Input: part model. Units: mm. Frame: model coordinates. A direction names the side the tool comes from. Coordinates: 2 decimals unless noted, no trailing zeros. Loops run counter-clockwise (first coordinate to the right, second up) from the corner with the lowest first, then second, coordinate; pieces in that order, holes last. Notation, with made-up numbers: (35, -29.5) - (80, -29.5) arc R34 cw to (80, 2.5) - close; hole circle Ø4 at (-4, 82). An arc over 180 degrees is marked (long way). Answer as CSV lines item,"result". Start each with the question number.
```python
from build123d import *

# Parameters (mm, degrees)
SKETCH_2_W          = 380.47
SKETCH_2_H          = 189.04
EXTRUDE_1_DEPTH     = 3
SKETCH_3_W          = 368.48
SKETCH_3_H          = 177.01
EXTRUDE_2_DEPTH     = 11.5
SKETCH_4_W          = 352.48
SKETCH_4_H          = 161.01
CUT_EXTRUDE_1_DEPTH = 11.5


with BuildPart() as part:
    # 草图2 → 凸台-拉伸1 (new body)
    with BuildSketch(Plane.XY):
        with Locations((183.815306963, 88.27515573)):
            Rectangle(SKETCH_2_W, SKETCH_2_H)
    extrude(amount=EXTRUDE_1_DEPTH)

    # 草图3 → 凸台-拉伸2 (add)
    with BuildSketch(Plane.XY.offset(3)):
        with Locations((183.815306963, 88.27515573)):
            Rectangle(SKETCH_3_W, SKETCH_3_H)
    extrude(amount=EXTRUDE_2_DEPTH)

    # 草图4 → 切除-拉伸1 (cut)
    with BuildSketch(Plane.XY.offset(14.5)):
        with Locations((183.815306963, 88.27515573)):
            Rectangle(SKETCH_4_W, SKETCH_4_H)
    extrude(amount=-CUT_EXTRUDE_1_DEPTH, mode=Mode.SUBTRACT)


solid = part.part
```
Item 1: Set-up query: faces 1 (the flat face through (181, 176.78, 9)), 2 (the flat face through (181, 168.78, 9)), 3 (the flat face through (-0.425, 87, 9)). Return all of +Z, -Z, +X, -X, +Y, -Y with unobstructed straight access to the full face (end or side cutting, diameter ignored); none if empty.
Item 2: Section query C-C, the plane x = 66.5. Output: boundary loops of the cut face in (y, z).
Item 3: Draft query along X for faces 4 (the flat face through (368.055, 87, 9)), 5 (the flat face through (181, 7.77, 9)), 6 (the flat face through (183, 180, 3)). Return one class per face: pulls with the +X half, pulls with the -X half, needs draft (parallel to the pull), parting line crosses it, or undercut.
Item 4: Section query A-A, the plane z = 8.5. Output: boundary loops of the cut face in (x, y), and give its area (3 significant figures).
Item 5: Contact query for flat-ended pins moving along their axis: P1, Ø10, axis at x = 150.5, y = 66.5, coming from the +Z side; P2, Ø1.5, axis at y = 59.5, z = 6.5, coming from the +X side; P3, Ø6, axis at x = 233.5, z = 10.5, coming from the +Y side. Output: stop coordinate, or through.
Item 6: Material intervals for probe 1 along X at (y, z) = (19, 4.5); probe 2 along Y at (x, z) = (195.5, 3.25); probe 3 along Z at (x, y) = (300, 158.5), sorted ascending.
Item 7: Section query B-B, the plane y = 113. Output: boundary loops of the cut face in (x, z), and give its area (3 significant figures).
Response values:
1,face 1,"+Z, +X, -X, +Y"
1,face 2,"+Z"
1,face 3,"+Z, -X, +Y, -Y"
2,outline,"(-6.24, 0) - (182.8, 0) - (182.8, 3) - (176.78, 3) - (176.78, 14.5) - (168.78, 14.5) - (168.78, 3) - (7.77, 3) - (7.77, 14.5) - (-0.23, 14.5) - (-0.23, 3) - (-6.24, 3) - close"
3,face 4,"pulls with the +X half"
3,face 5,"undercut"
3,face 6,"needs draft"
4,outline,"(-0.42, -0.23) - (368.06, -0.23) - (368.06, 176.78) - (-0.42, 176.78) - close; hole (7.58, 7.77) - (360.06, 7.77) - (360.06, 168.78) - (7.58, 168.78) - close"
4,area,"8,470 mm²"
5,P1,"stops at z = 3"
5,P2,"stops at x = 368.06"
5,P3,"stops at y = 176.78"
6,probe 1,"x = -0.42 to 7.58, 360.06 to 368.06"
6,probe 2,"y = -0.23 to 7.77, 168.78 to 176.78"
6,probe 3,"z = 0 to 3"
7,outline,"(-6.42, 0) - (374.05, 0) - (374.05, 3) - (368.06, 3) - (368.06, 14.5) - (360.06, 14.5) - (360.06, 3) - (7.58, 3) - (7.58, 14.5) - (-0.42, 14.5) - (-0.42, 3) - (-6.42, 3) - close"
7,area,"1,330 mm²"
